The listing builds one solid part. Answer for the finished solid, in the listing's coordinates (mm). Round coordinates to 2 decimals unless told otherwise and drop trailing zeros. Loops run counter-clockwise (first coordinate to the right, second up) from the corner with the lowest first, then second, coordinate; pieces in that order, holes last. Notation, with made-up numbers: (48, 9.5) - (87, 9.5) arc R13 ccw to (87, 21.5) - close; hole circle Ø7 at (61, -14.75). An arc over 180 degrees is marked (long way). Write item = value, one per line. Start each with the question number.
1) Section A-A, the plane z = 0 is taken. Determine the outline of the cut face in (x, y).
2) Section C-C, the plane x = 3.15 is taken. Give the number of separate pieces and of enclosed holes in the cut face, and give its area (3 significant figures).
3) For a pull along Y with two mould halves and no side action, classify faces 1 (the flat face through (0, 58, -1)), 2 (the flat face through (1.932, -10.456, 41.633)) as released by +Y, released by -Y, zero draft, split by the parting line, or undercut.
4) Given pin 1 Ø1 at (x, y) = (2, -34.5) entering from +Z; pin 2 Ø1 at (x, y) = (0.5, 41.5) entering from +Z, each flat-ended and moving along its own axis, determine where each tip first touches the part or whether it passes through.
5) Straight lines are drawn through the part: line 1 along Z through (x, y) = (2.8, -48); line 2 along Y through (x, z) = (3.35, 52); line 3 along Z through (x, y) = (0.9, -45.5). For each, find the intervals that lie inside material, in ascending order.
from build123d import *

# Parameters (mm, degrees)
SKETCH1_R           = 88.9
BOSS_EXTRUDE2_DEPTH = 3.81
CUT_EXTRUDE1_DEPTH  = 126.781302665
SKETCH4_R           = 4.445
CUT_EXTRUDE2_DEPTH  = 126.781302665
SKETCH5_R           = 3.81
CUT_EXTRUDE3_DEPTH  = 126.781302665


with BuildPart() as part:
    # Sketch1 → Boss-Extrude2 (new body)
    with BuildSketch(Plane(origin=(0, 0, 0), x_dir=(0, 0, -1), z_dir=(1, 0, 0))):
        with Locations(Location((0, 0, 0), (0, 0, 180))):
            Circle(SKETCH1_R)
    extrude(amount=BOSS_EXTRUDE2_DEPTH)

    # Sketch3 → Cut-Extrude1 (cut, through all)
    with BuildSketch(Plane(origin=(3.81, 0, 0), x_dir=(0, 0, -1), z_dir=(1, 0, 0))):
        with BuildLine():
            Line((9.320240363, 34.501930882), (11.560431238, 48.566486821))
            ThreePointArc((11.560431238, 48.566486821), (14.63716777, 53.055777419), (20.060305751, 53.513611663))
            ThreePointArc((20.060305751, 53.513611663), (40.411152545, 40.411152545), (53.513611663, 20.060305751))
            ThreePointArc((53.513611663, 20.060305751), (53.055777419, 14.63716777), (48.566486821, 11.560431238))
            Line((48.566486821, 11.560431238), (34.501930882, 9.320240363))
            ThreePointArc((34.501930882, 9.320240363), (32.819625412, 8.267039897), (32.408501994, 6.325298295))
            ThreePointArc((32.408501994, 6.325298295), (33.02, 0), (32.408501994, -6.325298295))
            ThreePointArc((32.408501994, -6.325298295), (32.819625412, -8.267039897), (34.501930882, -9.320240363))
            Line((34.501930882, -9.320240363), (48.566486821, -11.560431238))
            ThreePointArc((48.566486821, -11.560431238), (53.055777419, -14.63716777), (53.513611663, -20.060305751))
            ThreePointArc((53.513611663, -20.060305751), (40.411152545, -40.411152545), (20.060305751, -53.513611663))
            ThreePointArc((20.060305751, -53.513611663), (14.63716777, -53.055777419), (11.560431238, -48.566486821))
            Line((11.560431238, -48.566486821), (9.320240363, -34.501930882))
            ThreePointArc((9.320240363, -34.501930882), (8.267039897, -32.819625412), (6.325298295, -32.408501994))
            ThreePointArc((6.325298295, -32.408501994), (0, -33.02), (-6.325298295, -32.408501994))
            ThreePointArc((-6.325298295, -32.408501994), (-8.267039897, -32.819625412), (-9.320240363, -34.501930882))
            Line((-9.320240363, -34.501930882), (-11.560431238, -48.566486821))
            ThreePointArc((-11.560431238, -48.566486821), (-14.63716777, -53.055777419), (-20.060305751, -53.513611663))
            ThreePointArc((-20.060305751, -53.513611663), (-40.411152545, -40.411152545), (-53.513611663, -20.060305751))
            ThreePointArc((-53.513611663, -20.060305751), (-53.055777419, -14.63716777), (-48.566486821, -11.560431238))
            Line((-48.566486821, -11.560431238), (-34.501930882, -9.320240363))
            ThreePointArc((-34.501930882, -9.320240363), (-32.819625412, -8.267039897), (-32.408501994, -6.325298295))
            ThreePointArc((-32.408501994, -6.325298295), (-33.02, 0), (-32.408501994, 6.325298295))
            ThreePointArc((-32.408501994, 6.325298295), (-32.819625412, 8.267039897), (-34.501930882, 9.320240363))
            Line((-34.501930882, 9.320240363), (-48.566486821, 11.560431238))
            ThreePointArc((-48.566486821, 11.560431238), (-53.055777419, 14.63716777), (-53.513611663, 20.060305751))
            ThreePointArc((-53.513611663, 20.060305751), (-40.411152545, 40.411152545), (-20.060305751, 53.513611663))
            ThreePointArc((-20.060305751, 53.513611663), (-14.63716777, 53.055777419), (-11.560431238, 48.566486821))
            Line((-11.560431238, 48.566486821), (-9.320240363, 34.501930882))
            ThreePointArc((-9.320240363, 34.501930882), (-8.267039897, 32.819625412), (-6.325298295, 32.408501994))
            ThreePointArc((-6.325298295, 32.408501994), (0, 33.02), (6.325298295, 32.408501994))
            ThreePointArc((6.325298295, 32.408501994), (8.267039897, 32.819625412), (9.320240363, 34.501930882))
        make_face()
    extrude(amount=-CUT_EXTRUDE1_DEPTH, mode=Mode.SUBTRACT)

    # Sketch4 → Cut-Extrude2 (cut, through all)
    with BuildSketch(Plane.ZY):
        with Locations((0, 40.386)):
            Circle(SKETCH4_R)
        with Locations((40.386, 0)):
            Circle(SKETCH4_R)
        with Locations((0, -40.386)):
            Circle(SKETCH4_R)
        with Locations((-40.386, 0)):
            Circle(SKETCH4_R)
    extrude(amount=-CUT_EXTRUDE2_DEPTH, mode=Mode.SUBTRACT)

    # Sketch5 → Cut-Extrude3 (cut, through all)
    with BuildSketch(Plane(origin=(3.81, 0, 0), x_dir=(0, 0, -1), z_dir=(1, 0, 0))):
        with Locations((-12.7, 78.352413013)):
            Circle(SKETCH5_R)
        with Locations((-34.053975265, 64.598586623)):
            Circle(SKETCH5_R)
        with Locations((-49.624372091, 44.530633496)):
            Circle(SKETCH5_R)
        with Locations((70.593057135, 36.290644928)):
            Circle(SKETCH5_R)
        with Locations((50.913649668, 52.349316161)):
            Circle(SKETCH5_R)
        with Locations((27.01637485, 60.956304965)):
            Circle(SKETCH5_R)
        with Locations((56.328908679, -55.923560974)):
            Circle(SKETCH5_R)
        with Locations((65.520341251, -32.244929948)):
            Circle(SKETCH5_R)
        with Locations((66.321410001, -6.857565199)):
            Circle(SKETCH5_R)
        with Locations((-35.779877022, -70.853306382)):
            Circle(SKETCH5_R)
        with Locations((-10.41985182, -72.277778833)):
            Circle(SKETCH5_R)
        with Locations((13.972510712, -65.194513338)):
            Circle(SKETCH5_R)
        with Locations((-78.442088792, 12.133809414)):
            Circle(SKETCH5_R)
        with Locations((-71.960163834, -12.425194003)):
            Circle(SKETCH5_R)
        with Locations((-57.685923473, -33.434859923)):
            Circle(SKETCH5_R)
    extrude(amount=-CUT_EXTRUDE3_DEPTH, mode=Mode.SUBTRACT)


solid = part.part
Geometry check:
q1.outline = (0, -88.9) - (3.81, -88.9) - (3.81, -44.83) - (0, -44.83) - close; (0, -35.94) - (3.81, -35.94) - (3.81, -33.02) - (0, -33.02) - close; (0, 33.02) - (3.81, 33.02) - (3.81, 35.94) - (0, 35.94) - close; (0, 44.83) - (3.81, 44.83) - (3.81, 88.9) - (0, 88.9) - close
q2.separate_pieces = 1
q2.enclosed_holes = 20
q2.area = 15,800 mm2
q3.face_1 = zero draft
q3.face_2 = undercut
q4.pin_1 = 82.14
q4.pin_2 = 78.88
q5.line_1 = -74.83 to -31.02, -11.47 to 11.47, 31.02 to 74.83
q5.line_2 = -72.11 to -23.71, -13.28 to 13.28, 23.71 to 41.55, 47.51 to 72.11
q5.line_3 = -76.37 to -34.58, -11.07 to 11.07, 34.58 to 76.37
